Check sheet for the modelled part. Datum: model origin and axes. Units: mm. Face numbers are marked on the shaded views. A direction names the side the tool comes from. Give positions to 0.01 mm unless a question says otherwise; leave off trailing zeros. Order: outer loops, then holes, each group sorted by start corner. A loop starts at its lowest first (then second) coordinate and runs counter-clockwise, first axis right, second up.
from build123d import *

# Parameters (mm, degrees)
SKETCH_2_R          = 68.303668196
SKETCH_2_R_2        = 10.05
SKETCH_2_R_3        = 40.203668196
EXTRUDE_1_DEPTH     = 10
EXTRUDE_START       = -5
SKETCH_3_R          = 10.05
EXTRUDE_2_DEPTH     = 5
SKETCH_4_W          = 280.2912044
SKETCH_4_H          = 106.849461173
CUT_EXTRUDE_2_DEPTH = 45
SKETCH_5_R          = 2.1
CUT_EXTRUDE_3_DEPTH = 45
FILLET_1_R          = 10


with BuildPart() as part:
    # 草图2 → 凸台-拉伸1 (new body)
    with BuildSketch(Plane(origin=(0, 0, 0), x_dir=(1, 0, 0), z_dir=(0, 1, 0))):
        with Locations(Location((0, 0, 0), (0, 0, 270))):
            Circle(SKETCH_2_R)
        with Locations(Location((40, 36.653246961, 0), (0, 0, 270))):
            Circle(SKETCH_2_R_2, mode=Mode.SUBTRACT)
        with Locations(Location((0, 0, 0), (0, 0, 270))):
            Circle(SKETCH_2_R_3, mode=Mode.SUBTRACT)
        with Locations(Location((-40, 36.653246961, 0), (0, 0, 90))):
            Circle(SKETCH_2_R_2, mode=Mode.SUBTRACT)
    extrude(amount=EXTRUDE_1_DEPTH)

    # 草图3 → 凸台-拉伸2 (add)
    with BuildSketch(Plane(origin=(0, 10, 0), x_dir=(1, 0, 0), z_dir=(0, 1, 0)).offset(EXTRUDE_START)):
        with Locations(Location((-40, 36.653246961, 0), (0, 0, 90))):
            Circle(SKETCH_3_R)
        with Locations(Location((40, 36.653246961, 0), (0, 0, 270))):
            Circle(SKETCH_3_R)
    extrude(amount=EXTRUDE_2_DEPTH)

    # 草图4 → 切除-拉伸2 (cut)
    with BuildSketch(Plane(origin=(0, 0, 0), x_dir=(-1, 0, 0), z_dir=(0, -1, 0))):
        with Locations((7.276792676, -53.424730587)):
            Rectangle(SKETCH_4_W, SKETCH_4_H)
    extrude(amount=-CUT_EXTRUDE_2_DEPTH, mode=Mode.SUBTRACT)

    # 草图5 → 切除-拉伸3 (cut)
    with BuildSketch(Plane(origin=(0, 5, 0), x_dir=(-1, 0, 0), z_dir=(0, -1, 0))):
        with Locations(Location((-40, 41.653246961, 0), (0, 0, 90))):
            Circle(SKETCH_5_R)
        with Locations(Location((-35.669872981, 34.153246961, 0), (0, 0, 90))):
            Circle(SKETCH_5_R)
        with Locations(Location((-44.330127019, 34.153246961, 0), (0, 0, 90))):
            Circle(SKETCH_5_R)
    cut_extrude_3 = extrude(amount=-CUT_EXTRUDE_3_DEPTH, mode=Mode.SUBTRACT)

    # 镜向1: 切除-拉伸3 across plane
    add(cut_extrude_3.mirror(Plane(origin=(0, 0, 0), x_dir=(0, 0, 1), z_dir=(1, 0, 0))), mode=Mode.SUBTRACT)

    # 圆角1
    fillet_1_edges = [part.edges().sort_by_distance(p)[0] for p in [
        (-40.203668196, 5, 0),
        (40.203668196, 5, 0),
        (68.303668196, 5, 0),
        (-68.303668196, 5, 0),
    ]]
    fillet(fillet_1_edges, radius=FILLET_1_R)


solid = part.part
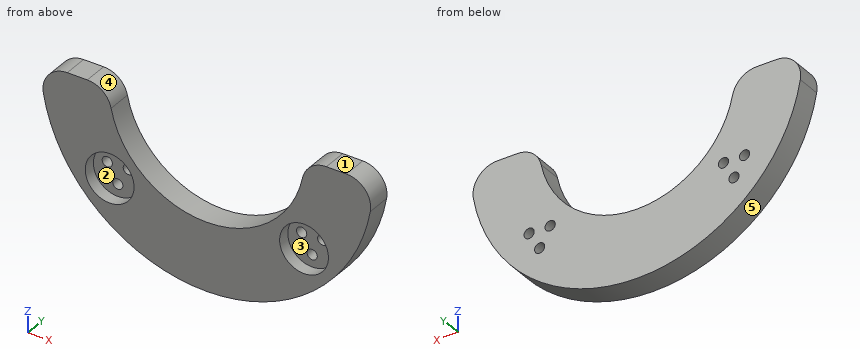
1) Section check B-B, the plane x = -27. Record the cut outline in (y, z).
Recorded:
outline: (0, -62.74) - (10, -62.74) - (10, -29.79) - (0, -29.79) - close
2) Draft check along Z on the marked faces 3, 4 and 5. Enter one of: +Z half, -Z half, draft (parallel to the pull), parting line (faces both ways), or undercut.
Recorded:
face 3: undercut
face 4: +Z half
face 5: -Z half
3) Material ranges on L1, parallel to X at y = 5.25, z = -46.5; L2, parallel to Y at x = -42.5, z = -39.5; L3, parallel to X at y = 7, z = -27, recorded low to high.
Recorded:
L1: x = -50.03 to 50.03
L2: y = 5 to 10
L3: x = -62.74 to -29.79, 29.79 to 62.74
4) Section check C-C, the plane z = -55. Record the cut outline in (x, y).
Recorded:
outline: (-40.5, 0) - (40.5, 0) - (40.5, 10) - (-40.5, 10) - close
5) Depth check by flat-ended pin: pin 1 Ø5 at (x, y) = (6.5, 6.5) entering from -Z; pin 2 Ø1 at (x, y) = (-8, 4.5) entering from +Z; pin 3 Ø5.5 at (x, z) = (-44.33, -34.15) entering from -Y; pin 4 Ø4 at (x, z) = (-40, -41.65) entering from +Y. Enter the tip coordinate at first touch or a pass-through.
Recorded:
pin 1: stops at z = -68.19
pin 2: stops at z = -39.29
pin 3: stops at y = 5
pin 4: passes through
6) Section check A-A, the plane y = 2. Record the cut outline in (x, z).
Recorded:
outline: (-67.29, -11.72) arc R68.3 ccw to (67.29, -11.72) arc R10 ccw to (57.44, 0) - (49.2, 0) arc R10 ccw to (39.4, -8.01) arc R40.2 cw to (-39.4, -8.01) arc R10 ccw to (-49.2, 0) - (-57.44, 0) arc R10 ccw to start; hole circle Ø20.1 at (-40, -36.65); hole circle Ø20.1 at (40, -36.65)
7) Set-up check for the marked faces 1 and 2: record each of +Z, -Z, +X, -X, +Y, -Y from which the full face is reachable in a straight line by a thin tool's end or side.
Recorded:
face 1: +Z, +X, -X, +Y, -Y
face 2: -Y
